Autodesk Inventor part; units mm, degrees
ref_plane "YZ Plane" through (0, 0, 0) normal (1, 0, 0) x (0, 1, 0)
ref_plane "XZ Plane" through (0, 0, 0) normal (0, 1, 0) x (-1, 0, 0)
ref_plane "XY Plane" through (0, 0, 0) normal (0, 0, 1) x (1, 0, 0)
sketch "Sketch1" plane through (0, 0, 0) normal (0, 1, 0) x (-1, 0, 0)
  line L0 (19.05, 47.498) -> (-19.05, 47.498)
  line L1 (-19.05, 47.498) -> (-19.05, -47.498)
  line L2 (-19.05, -47.498) -> (19.05, -47.498)
  line L3 (19.05, -47.498) -> (19.05, 47.498)
  line L4 (19.05, 47.498) -> (-19.05, -47.498) construction
  line L5 (-19.05, 47.498) -> (19.05, -47.498) construction
  point P0 (0, 0)
  dimension "d0" = 38.1
  dimension "d1" = 94.996
extrude "Extrusion1" add sketch "Sketch1" along normal blind 6.35
sketch "Sketch2" plane through (19.05, 0, 47.498) normal (1, 0, 0) x (0, 0, -1)
  line L0 (-35.052, 19.05) -> (130.048, 19.05)
  line L1 (130.048, 19.05) -> (130.048, 0)
  line L2 (130.048, 0) -> (-35.052, 0)
  line L3 (-35.052, 0) -> (-35.052, 19.05)
  line L4 (-35.052, 19.05) -> (130.048, 0) construction
  line L5 (130.048, 19.05) -> (-35.052, 0) construction
  line L6 (0, 0) -> (94.996, 0)
  circle A0 centre (-35.052, 9.525) radius 9.525
  circle A1 centre (130.048, 9.525) radius 9.525
  point P0 (47.498, 0)
  point P1 (47.498, 9.525)
  point P2 (47.498, 0)
  dimension "d4" = 165.1
  dimension "d5" = 19.05
extrude "Extrusion2" add sketch "Sketch2" against normal blind 6.35
fillet "Fillet1" radius 2.54 9 edges at (12.7, 0, -65.024) (12.7, 19.05, 0) (12.7, 9.525, 92.075) (12.7, 0, 65.024) (12.7, 9.525, -92.075) (19.05, 19.05, 0) (19.05, 9.525, 92.075) (19.05, 0, 0) (19.05, 9.525, -92.075)
mirror "Mirror1" about plane through (0, 0, 0) normal (1, 0, 0) of "Extrusion2", "Fillet1"
sketch "Sketch3" plane through (19.05, 9.525, 82.55) normal (1, 0, 0) x (0, 0, -1)
  arc A0 (165.1, -6.985) -> (165.1, 6.985) centre (165.1, 0) ccw
  point P0 (82.55, -9.525)
  point P1 (0, 0)
hole "Hole1" at (19.05, 9.525, 82.55) at (19.05, 9.525, -82.55) direction (-1, 0, 0) diameter 8.89 end through all
properties part number "Thin Leg"
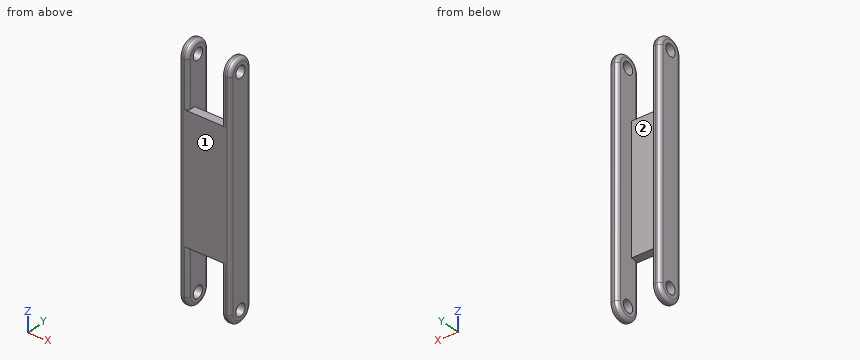
Design review of the part built by this model. Coordinates are the model's own, in mm. Face numbers are marked on the shaded views. Give positions to 0.01 mm unless a question says otherwise; leave off trailing zeros. Loops run counter-clockwise (first coordinate to the right, second up) from the corner with the lowest first, then second, coordinate; pieces in that order, holes last. Notation, with made-up numbers: (77.25, -1.75) -> (92.25, -1.75) arc R29 ccw to (92.25, 29.25) -> close; hole circle Ø10 at (67, 85.5). An arc over 180 degrees is marked (long way). One line per question, with ' | ' between items. Start each with the question number.
(1) We need section B-B (z = 20.5). State the section outline as (x, y) points, and give its area (3 significant figures).
(2) We need section C-C (x = 0). State the section outline as (y, z) points.
(3) Insertion check: P1, Ø10, axis at x = -3, z = -6.5, coming from the +Y side; P2, Ø7, axis at x = 1.5, y = 4.5, coming from the -Z side; P3, Ø8, axis at x = -10.5, y = 14, coming from the +Z side. Each pin has a flat end and moves straight along its axis. Give the tip position at first contact, or say it passes through.
(4) We need section A-A (z = 52). State the section outline as (x, y) points.
(5) We need section D-D (y = 12). State how many separate pieces and enclosed holes the cut face has, and give its area (3 significant figures).
(6) Draft analysis for pull direction X (two halves, no side actions). For the marked faces 1 and 2, state which applies: +X half, -X half, draft (parallel to the pull), parting line (faces both ways), or undercut.
(7) For line 1 (Y direction, x = -15.5, z = -82.55); line 2 (X direction, y = 16.25, z = -50.5); line 3 (Y direction, x = -14, z = 82), list the stretches that pass through material, from the lowest coordinate up.
The answers:
1) outline: (-19.05, 2.54) arc R2.54 ccw to (-16.51, 0) -> (16.51, 0) arc R2.54 ccw to (19.05, 2.54) -> (19.05, 16.51) arc R2.54 ccw to (16.51, 19.05) -> (15.24, 19.05) arc R2.54 ccw to (12.7, 16.51) -> (12.7, 6.35) -> (-12.7, 6.35) -> (-12.7, 16.51) arc R2.54 ccw to (-15.24, 19.05) -> (-16.51, 19.05) arc R2.54 ccw to (-19.05, 16.51) -> close | area: 395 mm^2
2) outline: (0, -47.5) -> (6.35, -47.5) -> (6.35, 47.5) -> (0, 47.5) -> close
3) P1: stops at y = 6.35 | P2: stops at z = -47.5 | P3: stops at z = 91.4
4) outline: (-19.05, 2.54) arc R2.54 ccw to (-16.51, 0) -> (-15.24, 0) arc R2.54 ccw to (-12.7, 2.54) -> (-12.7, 16.51) arc R2.54 ccw to (-15.24, 19.05) -> (-16.51, 19.05) arc R2.54 ccw to (-19.05, 16.51) -> close; (12.7, 2.54) arc R2.54 ccw to (15.24, 0) -> (16.51, 0) arc R2.54 ccw to (19.05, 2.54) -> (19.05, 16.51) arc R2.54 ccw to (16.51, 19.05) -> (15.24, 19.05) arc R2.54 ccw to (12.7, 16.51) -> close
5) separate pieces: 6 | enclosed holes: 0 | area: 2,130 mm^2
6) face 1: draft | face 2: undercut
7) line 1: y = 0 to 5.08, 13.97 to 19.05 | line 2: x = -19.05 to -12.7, 12.7 to 19.05 | line 3: y = 0.32 to 5.11, 13.94 to 18.73
